Design review of the part built by this model. Coordinates are the model's own, in mm. Give positions to 0.01 mm unless a question says otherwise; leave off trailing zeros. Order: outer loops, then holes, each group sorted by start corner. A loop starts at its lowest first (then second) coordinate and runs counter-clockwise, first axis right, second up. Notation, with made-up numbers: (-39.5, 71) -> (17.5, 71) arc R3 ccw to (17.5, 75) -> close; hole circle Ø1 at (-24.75, 64.5). An arc over 180 degrees is marked (long way). Return JSON: item names as keys, results as strings.
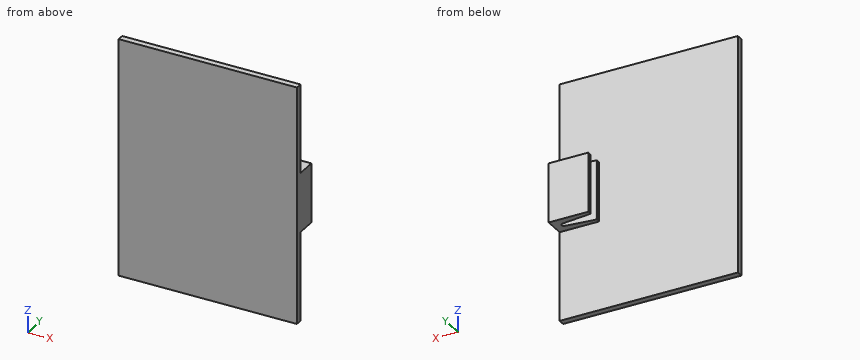
```python
from build123d import *

# Parameters (mm, degrees)
SKETCH1_W               = 450
SKETCH1_H               = 600
BOSS_EXTRUDE1_DEPTH     = 16
SKETCH2_W               = 100
SKETCH2_H               = 150
BOSS_EXTRUDE2_DEPTH     = 50
CUT_EXTRUDE1_DEPTH      = 443.273670932
CUT_EXTRUDE1_DEPTH_BACK = 443.273670932


with BuildPart() as part:
    # Sketch1 → Boss-Extrude1 (new body)
    with BuildSketch(Plane(origin=(0, 0, 0), x_dir=(1, 0, 0), z_dir=(0, 1, 0))):
        Rectangle(SKETCH1_W, SKETCH1_H)
    extrude(amount=BOSS_EXTRUDE1_DEPTH)

    # Sketch2 → Boss-Extrude2 (add)
    with BuildSketch(Plane(origin=(0, 16, 0), x_dir=(1, 0, 0), z_dir=(0, 1, 0))):
        with Locations((175, 0)):
            Rectangle(SKETCH2_W, SKETCH2_H)
    extrude(amount=BOSS_EXTRUDE2_DEPTH)

    # Sketch3 → Cut-Extrude1 (cut, two sides: drawn at the far end of the back side and taken through both)
    with BuildSketch(Plane(origin=(0, 0, -75), x_dir=(-1, 0, 0), z_dir=(0, 0, -1)).offset(-CUT_EXTRUDE1_DEPTH_BACK)):
        with BuildLine():
            Line((-200.674344807, 46.961984492), (-126.621721722, 55.337887164))
            ThreePointArc((-126.621721722, 55.337887164), (-110.57068991, 41), (-126.621721722, 26.662112836))
            Line((-126.621721722, 26.662112836), (-200.674344807, 35.038015508))
            ThreePointArc((-200.674344807, 35.038015508), (-206, 41), (-200.674344807, 46.961984492))
        make_face()
    extrude(amount=CUT_EXTRUDE1_DEPTH + CUT_EXTRUDE1_DEPTH_BACK, mode=Mode.SUBTRACT)


solid = part.part
```
Item 1: Wall thickness on L1, parallel to Y at x = 30, z = 148; L2, parallel to Z at x = 204.5, y = 20; L3, parallel to X at y = 44, z = -74: over which ranges is each line inside the solid? List them lowest first. Write a range as [from, to].
Result set:
{"L1": "y = [0, 16]", "L2": "z = [-75, 75]", "L3": "x = [205.2, 225]"}
Item 2: For pin 1 (5.5 mm diameter, centred on y = 23.5, z = -35.5, fed in from -X); pin 2 (1 mm diameter, centred on x = 49, z = 92, fed in from +Y), all flat-tipped, find the tip position at first contact; note any pin that passes through.
Result set:
{"pin 1": "stops at x = 125", "pin 2": "stops at y = 16"}
Item 3: Add section B-B (x = 146). Give the boundary of the cut face in (y, z).
Result set:
{"outline": "(0, -300) -> (16, -300) -> (16, -75) -> (28.85, -75) -> (28.85, 75) -> (16, 75) -> (16, 300) -> (0, 300) -> close; (53.15, -75) -> (66, -75) -> (66, 75) -> (53.15, 75) -> close"}
Item 4: Add section D-D (z = -255). Give the boundary of the cut face in (x, y).
Result set:
{"outline": "(-225, 0) -> (225, 0) -> (225, 16) -> (-225, 16) -> close"}
Item 5: Add section A-A (z = -4). Give the boundary of the cut face in (x, y), plus the area to 3 significant figures.
Result set:
{"outline": "(-225, 0) -> (225, 0) -> (225, 66) -> (125, 66) -> (125, 55.43) arc R14.43 cw to (126.62, 55.34) -> (200.67, 46.96) arc R6 cw to (200.67, 35.04) -> (126.62, 26.66) arc R14.43 cw to (125, 26.57) -> (125, 16) -> (-225, 16) -> close", "area": "10,600 mm^2"}
Item 6: Add section C-C (x = -168). Give the boundary of the cut face in (y, z), plus the area to 3 significant figures.
Result set:
{"outline": "(0, -300) -> (16, -300) -> (16, 300) -> (0, 300) -> close", "area": "9,600 mm^2"}
